Check sheet for the drawn part. Datum: minimum x, y, z corner. Units: mm. A direction names the side the tool comes from. Coordinates: 2 decimals unless noted, no trailing zeros. Write each loop counter-clockwise with the first axis right and the second up, starting at its lowest first coordinate (ties: lowest second). Pieces come first, ordered by that corner, then holes. Notation, with made-up numbers: (4.5, 22.25) -> (55.5, 22.25) arc R12 cw to (55.5, 35.25) -> close; hole circle Ø5 at (70, -3). An arc over 180 degrees is marked (long way). Answer in a Markdown table with one row per item.
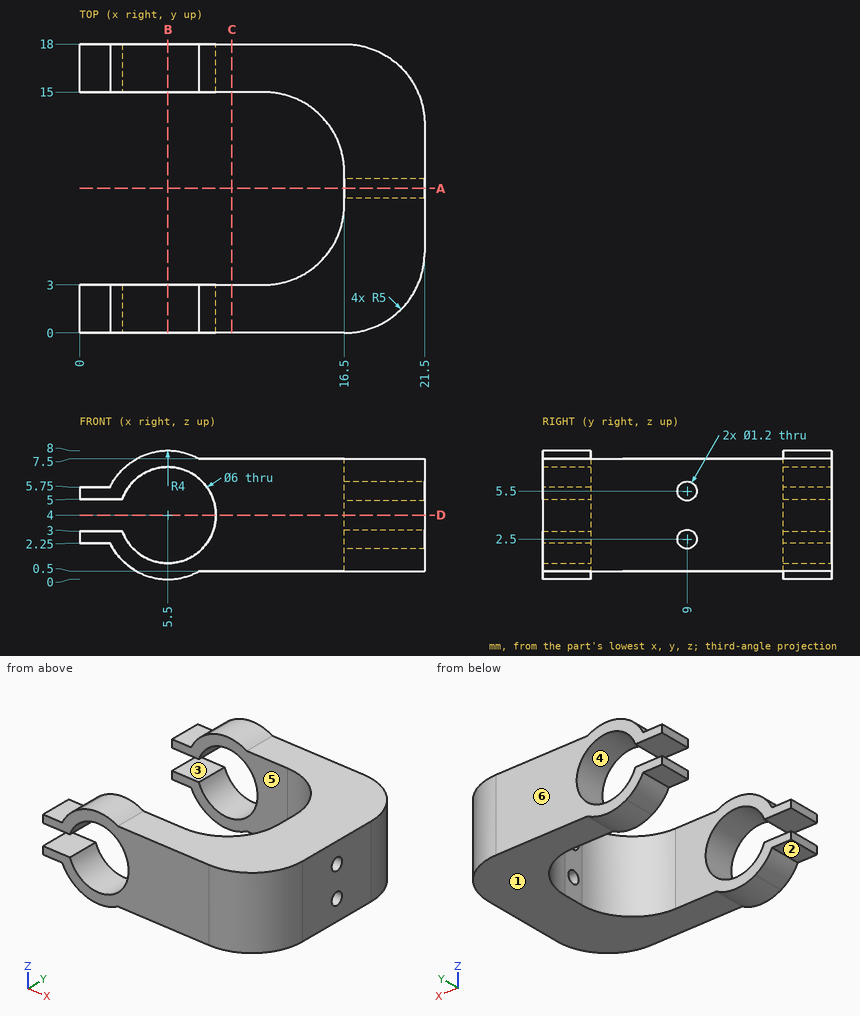
1. Release check for a two-part mould opening along Y. For the marked faces 4, 5 and 6 record: released by +Y, released by -Y, zero draft, split by the parting line, or undercut.
Findings below:
| item | result |
|---|---|
| face 4 | zero draft |
| face 5 | undercut |
| face 6 | released by +Y |
2. Go/stop test with flat-tipped pins: pin 1 (7 mm diameter, centred on x = 16.5, y = 12, fed in from +Z); pin 2 (1.5 mm diameter, centred on x = 1, y = 16, fed in from +Z); pin 3 (0.6 mm diameter, centred on y = 8.5, z = 5.5, fed in from -X); pin 4 (1.1 mm diameter, centred on y = 9, z = 2.5, fed in from +X). Record where each tip stops, or that it passes through.
Findings below:
| item | result |
|---|---|
| pin 1 | stops at z = 7.5 |
| pin 2 | stops at z = 5.75 |
| pin 3 | stops at x = 16.5 |
| pin 4 | passes through |
3. Material ranges on probe 1 along Y at (x, z) = (9.75, 4.5); probe 2 along Y at (x, z) = (16, 4.75); probe 3 along Z at (x, y) = (7.75, 1.5), recorded low to high. Write a range as from..to.
Findings below:
| item | result |
|---|---|
| probe 1 | y = 0..3, 15..18 |
| probe 2 | y = 0..5.82, 12.18..18 |
| probe 3 | z = 0.5..2.02, 5.98..7.5 |
4. Sectioned sample at A-A, the plane y = 9. Record the cut outline in (x, z), and give its area (3 significant figures).
Findings below:
| item | result |
|---|---|
| outline | (16.5, 0.5) -> (21.5, 0.5) -> (21.5, 1.9) -> (16.5, 1.9) -> close; (16.5, 3.1) -> (21.5, 3.1) -> (21.5, 4.9) -> (16.5, 4.9) -> close; (16.5, 6.1) -> (21.5, 6.1) -> (21.5, 7.5) -> (16.5, 7.5) -> close |
| area | 23.0 mm² |
5. Sectioned sample at D-D, the plane z = 4. Record the cut outline in (x, y).
Findings below:
| item | result |
|---|---|
| outline | (8.5, 0) -> (16.5, 0) arc R5 ccw to (21.5, 5) -> (21.5, 13) arc R5 ccw to (16.5, 18) -> (8.5, 18) -> (8.5, 15) -> (11.5, 15) arc R5 cw to (16.5, 10) -> (16.5, 8) arc R5 cw to (11.5, 3) -> (8.5, 3) -> close |
6. Sectioned sample at C-C, the plane x = 9.5. Record the cut outline in (y, z), and give its area (3 significant figures).
Findings below:
| item | result |
|---|---|
| outline | (0, 0.5) -> (3, 0.5) -> (3, 7.5) -> (0, 7.5) -> close; (15, 0.5) -> (18, 0.5) -> (18, 7.5) -> (15, 7.5) -> close |
| area | 42.0 mm² |
7. Access from +Z, -Z, +X, -X, +Y, -Y to the whole of each face (thin tool, end or side, straight path). Record for the marked faces 1, 2 and 3.
Findings below:
| item | result |
|---|---|
| face 1 | -Z, +X, +Y, -Y |
| face 2 | -Z, -X, +Y, -Y |
| face 3 | -X, +Y, -Y |
8. Sectioned sample at B-B, the plane x = 5.5. Record the cut outline in (y, z), and give its area (3 significant figures).
Findings below:
| item | result |
|---|---|
| outline | (0, 0) -> (3, 0) -> (3, 1) -> (0, 1) -> close; (0, 7) -> (3, 7) -> (3, 8) -> (0, 8) -> close; (15, 0) -> (18, 0) -> (18, 1) -> (15, 1) -> close; (15, 7) -> (18, 7) -> (18, 8) -> (15, 8) -> close |
| area | 12.0 mm² |
